Geometry check sheet. Reference: drawing and pictorial views, mm from the part's lowest x, y, z. Round coordinates to 2 decimals unless told otherwise and drop trailing zeros. Order: outer loops, then holes, each group sorted by start corner. A loop starts at its lowest first (then second) coordinate and runs counter-clockwise, first axis right, second up.
Q1. Mould release check, pull along X, two halves, no side actions. Record for the marked faces 1, 2 and 3: +X half, -X half, draft (parallel to the pull), parting line (faces both ways), or undercut.
Q2. Cross-section at C-C on y = 2.75. Record the cut outline in (x, z), then the cut area to 3 significant figures.
Q3. Cross-section at B-B on x = 25. Record the cut outline in (y, z).
Q4. Cross-section at A-A on z = 29.5. Record the cut outline in (x, y).
Q5. Scan lines: probe 1 along X at (y, z) = (5, 25); probe 2 along Z at (x, y) = (33, 2.5). Record each from-to range of solid material in increasing order.
Q6. Cross-section at D-D on x = 17. Record the cut outline in (y, z).
Q7. Depth check by flat-ended pin: P1, Ø2.5, axis at x = 25, z = 17, coming from the -Y side. Enter the tip coordinate at first touch or a pass-through.
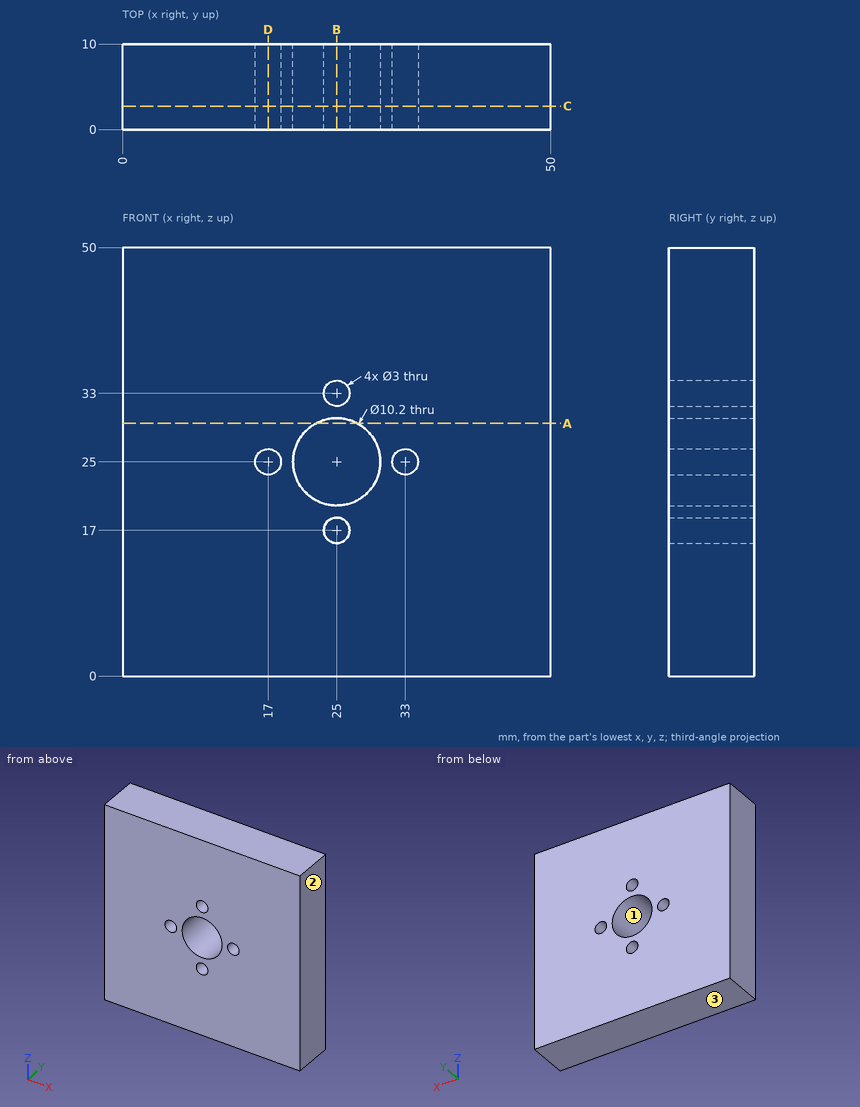
Results found:
1. face 1: undercut
1. face 2: +X half
1. face 3: draft
2. outline: (0, 0) - (50, 0) - (50, 50) - (0, 50) - close; hole circle Ø3 at (17, 25); hole circle Ø10.2 at (25, 25); hole circle Ø3 at (25, 17); hole circle Ø3 at (25, 33); hole circle Ø3 at (33, 25)
2. area: 2,390 mm2
3. outline: (0, 0) - (10, 0) - (10, 15.5) - (0, 15.5) - close; (0, 18.5) - (10, 18.5) - (10, 19.9) - (0, 19.9) - close; (0, 30.1) - (10, 30.1) - (10, 31.5) - (0, 31.5) - close; (0, 34.5) - (10, 34.5) - (10, 50) - (0, 50) - close
4. outline: (0, 0) - (22.6, 0) - (22.6, 10) - (0, 10) - close; (27.4, 0) - (50, 0) - (50, 10) - (27.4, 10) - close
5. probe 1: x = 0 to 15.5, 18.5 to 19.9, 30.1 to 31.5, 34.5 to 50
5. probe 2: z = 0 to 23.5, 26.5 to 50
6. outline: (0, 0) - (10, 0) - (10, 23.5) - (0, 23.5) - close; (0, 26.5) - (10, 26.5) - (10, 50) - (0, 50) - close
7. P1: passes through
